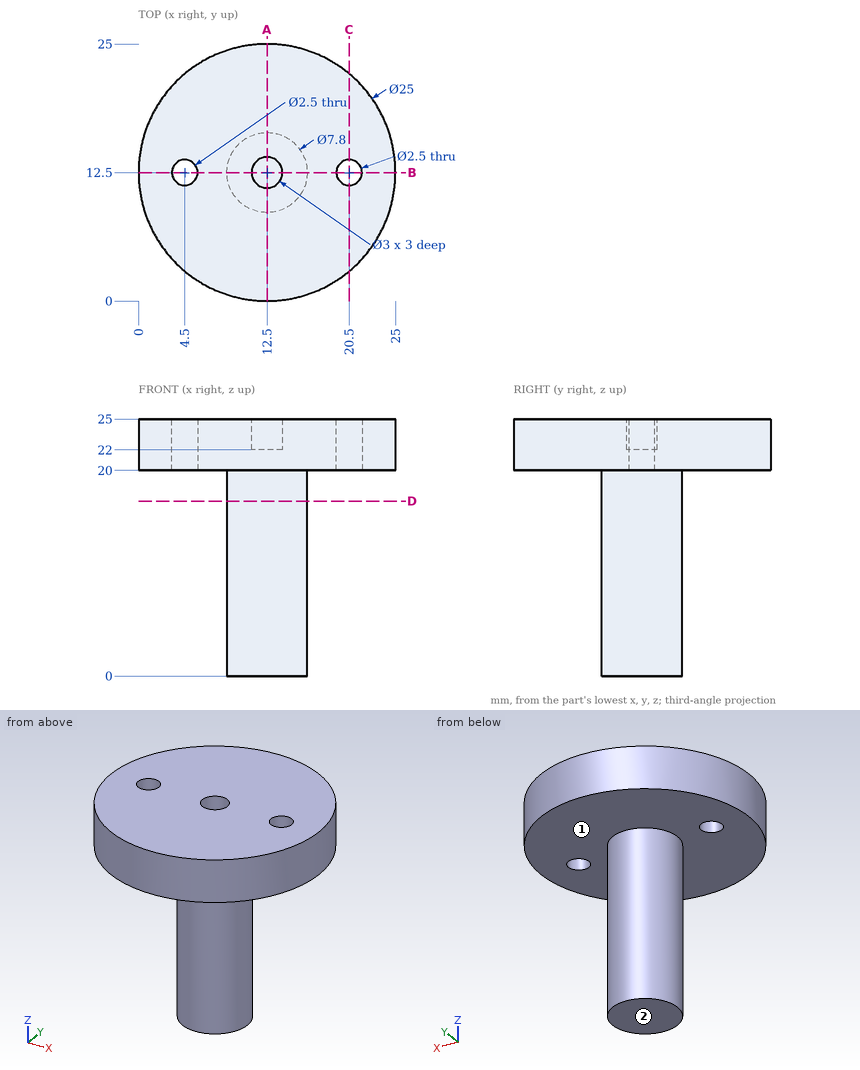
Part print with two shaded views. Sizes in mm from the minimum x, y, z corner. A direction names the side the tool comes from. Give positions to 0.01 mm unless a question says otherwise; leave off trailing zeros. Order: outer loops, then holes, each group sorted by start corner. A loop starts at its lowest first (then second) coordinate and runs counter-clockwise, first axis right, second up.
(1) Tool access for the marked faces 1 and 2: list every direction of +Z, -Z, +X, -X, +Y, -Y with a clear straight run to the whole face (end or side of a thin tool).
(2) Flat gauge pins, fed straight in: pin 1 (3 mm diameter, centred on x = 20.5, y = 12.5, fed in from +Z); pin 2 (3 mm diameter, centred on y = 16.5, z = 9, fed in from +X); pin 3 (1 mm diameter, centred on y = 8, z = 4, fed in from -X); pin 4 (5 mm diameter, centred on y = 5.5, z = 21.5, fed in from -X). Where does each tip first touch, or does it go through?
(3) Saw through at B-B, the plane y = 12.5. Give the cut face in (x, z).
(4) Saw through at D-D, the plane z = 17. Give the cut face in (x, y), then the cut area to 3 significant figures.
(5) Drill centre lines: L1, parallel to Z at x = 9, y = 5.75; L2, parallel to Y at x = 12.5, z = 23.8; L3, parallel to Y at x = 3.5, z = 20.25. Where is each one in solid material? Low to high.
(6) Saw through at A-A, the plane x = 12.5. Give the cut face in (y, z), then the cut area to 3 significant figures.
(7) Saw through at C-C, the plane x = 20.5. Give the cut face in (y, z), then the cut area to 3 significant figures.
Results found:
1. face 1: -Z
1. face 2: -Z, +X, -X, +Y, -Y
2. pin 1: stops at z = 25
2. pin 2: stops at x = 15.49
2. pin 3: passes through
2. pin 4: stops at x = 0.84
3. outline: (0, 20) - (3.25, 20) - (3.25, 25) - (0, 25) - close; (5.75, 20) - (8.6, 20) - (8.6, 0) - (16.4, 0) - (16.4, 20) - (19.25, 20) - (19.25, 25) - (14, 25) - (14, 22) - (11, 22) - (11, 25) - (5.75, 25) - close; (21.75, 20) - (25, 20) - (25, 25) - (21.75, 25) - close
4. outline: circle Ø7.8 at (12.5, 12.5)
4. area: 47.8 mm2
5. L1: z = 20 to 25
5. L2: y = 0 to 11, 14 to 25
5. L3: y = 3.83 to 11.75, 13.25 to 21.17
6. outline: (0, 20) - (8.6, 20) - (8.6, 0) - (16.4, 0) - (16.4, 20) - (25, 20) - (25, 25) - (14, 25) - (14, 22) - (11, 22) - (11, 25) - (0, 25) - close
6. area: 272 mm2
7. outline: (2.9, 20) - (11.25, 20) - (11.25, 25) - (2.9, 25) - close; (13.75, 20) - (22.1, 20) - (22.1, 25) - (13.75, 25) - close
7. area: 83.5 mm2
